Drawing for the job (mm, zero at the part's lowest x, y, z). A direction names the side the tool comes from. Coordinates: 2 decimals unless noted, no trailing zeros. Order: outer loops, then holes, each group sorted by start corner. A loop starts at its lowest first (then second) coordinate and runs counter-clockwise, first axis right, second up.
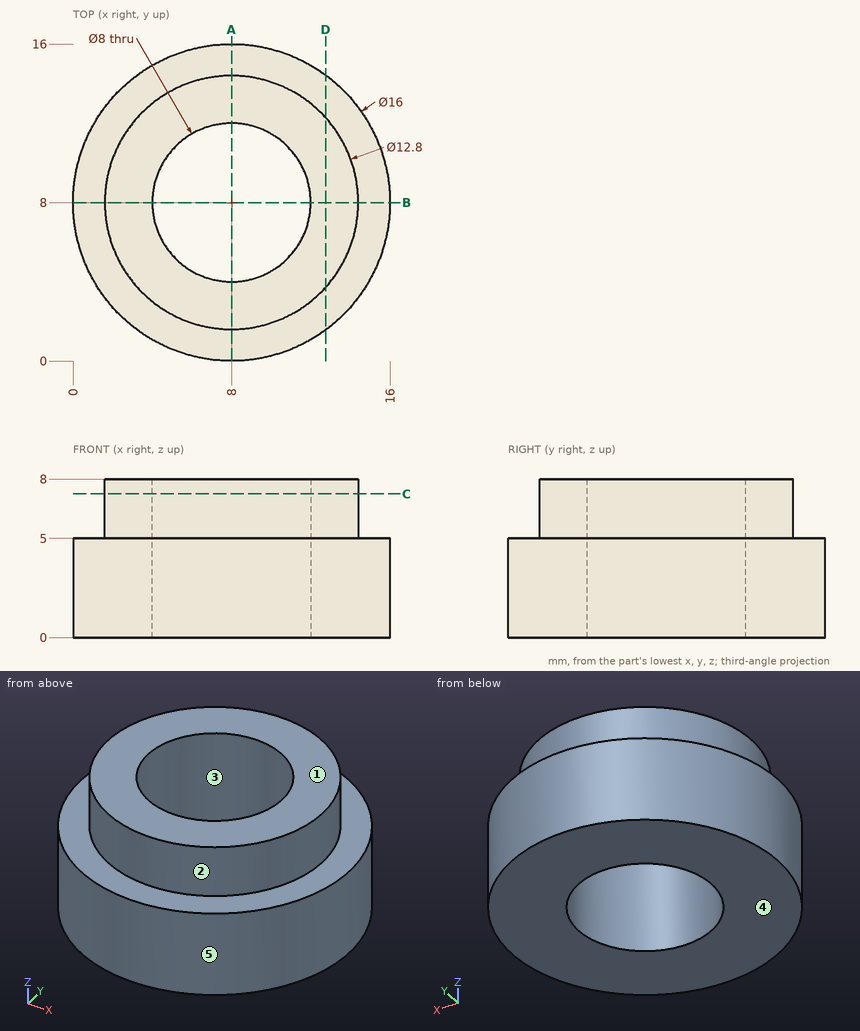
1) Slice it at A-A (x = 8). List the corners of the cut face in (y, z), plus the area to 3 significant figures.
2) Which spindle directions (+Z, -Z, +X, -X, +Y, -Y) get a long thin tool onto all of the face, cutting with end or side? Do the marked faces 1 and 2. Say none if no direction does.
3) Slice it at C-C (z = 7.25). List the corners of the cut face in (x, y).
4) Two-plate mould, pull along Y, no slides. Class the marked faces 3, 4 and 5: released by +Y, released by -Y, zero draft, split by the parting line, or undercut.
5) Pin check, flat tips, straight feed: P1, Ø1, axis at y = 9.5, z = 3, coming from the +X side; P2, Ø2, axis at y = 11, z = 3.5, coming from the +X side. Stop position of each tip, or through.
6) Drill centre lines: probe 1 along Y at (x, z) = (8, 6.25); probe 2 along Z at (x, y) = (2, 13); probe 3 along Y at (x, z) = (8, 2.75). Where is each one in solid material? Low to high.
7) Slice it at D-D (x = 12.75). List the corners of the cut face in (y, z), plus the area to 3 significant figures.
Worked out:
1. outline: (0, 0) - (4, 0) - (4, 8) - (1.6, 8) - (1.6, 5) - (0, 5) - close; (12, 0) - (16, 0) - (16, 5) - (14.4, 5) - (14.4, 8) - (12, 8) - close
1. area: 54.4 mm2
2. face 1: +Z, +X, -X, +Y, -Y
2. face 2: +Z
3. outline: circle Ø12.8 at (8, 8); hole circle Ø8 at (8, 8)
4. face 3: undercut
4. face 4: zero draft
4. face 5: split by the parting line
5. P1: stops at x = 15.94
5. P2: stops at x = 15.75
6. probe 1: y = 1.6 to 4, 12 to 14.4
6. probe 2: z = 0 to 5
6. probe 3: y = 0 to 4, 12 to 16
7. outline: (1.56, 0) - (14.44, 0) - (14.44, 5) - (12.29, 5) - (12.29, 8) - (3.71, 8) - (3.71, 5) - (1.56, 5) - close
7. area: 90.1 mm2
